Build history of the part. All positions in model axes, mm. Face numbers are marked on the shaded views. A direction names the side the tool comes from. Round coordinates to 2 decimals unless told otherwise and drop trailing zeros. Order: outer loops, then holes, each group sorted by start corner. A loop starts at its lowest first (then second) coordinate and runs counter-clockwise, first axis right, second up. Notation, with made-up numbers: (-37.75, 80) -> (-9.75, 80) arc R25 ccw to (-9.75, 102) -> close; hole circle Ø2 at (19.5, -38.75). An arc over 180 degrees is marked (long way). Answer as a JSON object with one key per item and string values.
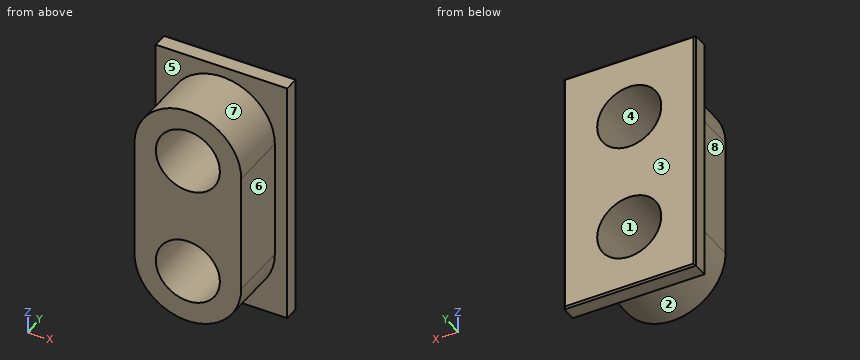
Autodesk Inventor part; units mm, degrees
ref_plane "YZ Plane" through (0, 0, 0) normal (1, 0, 0) x (0, 1, 0)
ref_plane "XZ Plane" through (0, 0, 0) normal (0, 1, 0) x (-1, 0, 0)
ref_plane "XY Plane" through (0, 0, 0) normal (0, 0, 1) x (1, 0, 0)
sketch "Skizze1" plane through (0, 0, 0) normal (0, 1, 0) x (-1, 0, 0)
  line L0 (0, 0) -> (80, 0)
  line L1 (80, 0) -> (80, -150)
  line L2 (80, -150) -> (0, -150)
  line L3 (0, -150) -> (0, 0)
  dimension "d0" = 80
  dimension "d1" = 150
extrude "Extrusion1" add sketch "Skizze1" along normal blind 10
sketch "Skizze2" plane through (0, 10, 0) normal (0, 1, 0) x (1, 0, 0)
  circle A0 centre (-40, 39) radius 19.5
  line L0 (-80, 0) -> (0, 0)
  line L1 (0, 150) -> (-80, 150)
  line L2 (-80, 150) -> (-80, 0)
  line L3 (-80, 75) -> (0, 75)
  circle A1 centre (-40, 111) radius 19.5
  dimension "d4" = 39
  dimension "d5" = 72
extrude "Extrusion2" cut sketch "Skizze2" against normal blind 10
sketch "Skizze3" plane through (0, 0, 0) normal (0, -1, 0) x (1, 0, 0)
  circle A0 centre (-40, -111) radius 19.5
  circle A1 centre (-40, -39) radius 19.5
  line L0 (-40, -111) -> (-40, -39) construction
  line L1 (-7.5, -111) -> (-7.5, -39)
  line L2 (-72.5, -39) -> (-72.5, -111)
  arc A2 (-72.5, -111) -> (-7.5, -111) centre (-40, -111) ccw
  arc A3 (-7.5, -39) -> (-72.5, -39) centre (-40, -39) ccw
  point P0 (0, 0)
  point P1 (-40, -75)
  dimension "d8" = 65
extrude "Extrusion3" add sketch "Skizze3" along normal blind 36
chamfer "Fasen1" distance 1 angle 45 4 edges at (-80, 10, -75) (-40, 10, -150) (0, 10, -75) (-40, 10, 0)
properties part number "Double_Steckdose" material "Gummi"
1) Cut at A-A, the plane x = -40. Give the cut face in (y, z), plus the area to 3 significant figures.
Checked values:
{"outline": "(-36, -143.5) -> (0, -143.5) -> (0, -150) -> (9, -150) -> (10, -149) -> (10, -130.5) -> (-36, -130.5) -> close; (-36, -91.5) -> (10, -91.5) -> (10, -58.5) -> (-36, -58.5) -> close; (-36, -19.5) -> (10, -19.5) -> (10, -1) -> (9, 0) -> (0, 0) -> (0, -6.5) -> (-36, -6.5) -> close", "area": "2,840 mm²"}
2) Pull direction Z, two halves, no side cores. Call the marked faces 1, 2, 3 and 4: pulls with the +Z half, pulls with the -Z half, needs draft (parallel to the pull), parting line crosses it, or undercut.
Checked values:
{"face 1": "undercut", "face 2": "pulls with the -Z half", "face 3": "needs draft", "face 4": "undercut"}
3) Probe L1, parallel to X at y = -3, z = -38.5; L2, parallel to Z at x = -38.5, y = -31; L3, parallel to Z at x = -35.5, y = -1. List the from-to ranges inside material, lowest first. Write a range as from..to.
Checked values:
{"L1": "x = -72.5..-59.49, -20.51..-7.5", "L2": "z = -143.47..-130.44, -91.56..-58.44, -19.56..-6.53", "L3": "z = -143.19..-129.97, -92.03..-57.97, -20.03..-6.81"}
4) Which spindle directions (+Z, -Z, +X, -X, +Y, -Y) get a long thin tool onto all of the face, cutting with end or side? Do the marked faces 5, 6, 7 and 8. Say none if no direction does.
Checked values:
{"face 5": "-Y", "face 6": "+Z, -Z, +X, -Y", "face 7": "+Z, -Y", "face 8": "+Z, -Z, -X, -Y"}
5) Cut at C-C, the plane y = -32.5. Give the cut face in (x, z).
Checked values:
{"outline": "(-72.5, -111) arc R32.5 ccw to (-7.5, -111) -> (-7.5, -39) arc R32.5 ccw to (-72.5, -39) -> close; hole circle Ø39 at (-40, -111); hole circle Ø39 at (-40, -39)"}
6) Cut at D-D, the plane x = -62.5. Give the cut face in (y, z), plus the area to 3 significant figures.
Checked values:
{"outline": "(-36, -134.45) -> (0, -134.45) -> (0, -150) -> (9, -150) -> (10, -149) -> (10, -1) -> (9, 0) -> (0, 0) -> (0, -15.55) -> (-36, -15.55) -> close", "area": "5,780 mm²"}
7) Cut at B-B, the plane z = -80.5. Give the cut face in (x, y).
Checked values:
{"outline": "(-80, 0) -> (-72.5, 0) -> (-72.5, -36) -> (-7.5, -36) -> (-7.5, 0) -> (0, 0) -> (0, 9) -> (-1, 10) -> (-79, 10) -> (-80, 9) -> close"}
8) Flat gauge pins, fed straight in: pin 1 Ø18 at (y, z) = (-19, -72.5) entering from -X; pin 2 Ø1.5 at (x, y) = (-14.5, -6) entering from -Z; pin 3 Ø6 at (y, z) = (-4.5, -18) entering from +X. Where does each tip first touch, or does it go through?
Checked values:
{"pin 1": "stops at x = -72.5", "pin 2": "stops at z = -132.06", "pin 3": "stops at x = -12.94"}
